from build123d import *

# Parameters (mm, degrees)
BOSS_EXTRUDE1_DEPTH = 6


with BuildPart() as part:
    # Sketch1 → Boss-Extrude1 (new body)
    with BuildSketch(Plane.XY):
        Polygon((20, -35), (20, 35), (10, 45), (10, 51), (-10, 51), (-10, 45), (-20, 35), (-20, -35), (-10, -45), (-10, -51), (10, -51), (10, -45), align=None)
        Polygon((5.757359313, 40.757359313), (15.757359313, 30.757359313), (15.757359313, -30.757359313), (5.757359313, -40.757359313), (-5.757359313, -40.757359313), (-15.757359313, -30.757359313), (-15.757359313, 30.757359313), (-5.757359313, 40.757359313), align=None, mode=Mode.SUBTRACT)
    extrude(amount=BOSS_EXTRUDE1_DEPTH)


solid = part.part
Check sheet for the modelled part. Datum: model origin and axes. Units: mm. A direction names the side the tool comes from. Give positions to 0.01 mm unless a question says otherwise; leave off trailing zeros. Write each loop counter-clockwise with the first axis right and the second up, starting at its lowest first coordinate (ties: lowest second). Pieces come first, ordered by that corner, then holes. Notation, with made-up numbers: (34, -36.75) -> (40, -36.75) arc R6 ccw to (40, -26.75) -> close; hole circle Ø6 at (70.25, 84.25). An arc over 180 degrees is marked (long way). Use one line per item in the form item = value. Start each with the question number.
1. Access from +Z, -Z, +X, -X, +Y, -Y to the whole of each face (thin tool, end or side, straight path). Record for faces 4 (the flat face through (-10, 48, 3)), 5 (the flat face through (10, 48, 3)), 6 (the flat face through (0, -51, 3)), 7 (the flat face through (-20, 0, 3)), 8 (the flat face through (-10.687, -35.827, 2.958)).
2. Section check C-C (y = 15). Record the cut outline in (x, z).
3. Section check A-A (z = 1.75). Record the cut outline in (x, y), and give its area (3 significant figures).
4. Mould release check, pull along Y, two halves, no side actions. Record for faces 1 (the flat face through (10, -48, 3)), 2 (the flat face through (-15, -40, 3)), 3 (the flat face through (15.757, 0, 3)): pulls with the +Y half, pulls with the -Y half, needs draft (parallel to the pull), parting line crosses it, or undercut.
5. Go/stop test with flat-tipped pins: P1, Ø12, axis at x = 8.5, y = -4.5, coming from the +Z side; P2, Ø1.8, axis at y = -47, z = 4.5, coming from the -X side. Record where each tip stops, or that it passes through.
6. Section check B-B (x = 3.5). Record the cut outline in (y, z), and give its area (3 significant figures).
7. Thickness scan on line 1 along Y through (x, z) = (0, 2.15); line 2 along X through (y, z) = (-14.5, 2.25); line 3 along Y through (x, z) = (-8, 5.5). Record the ranges inside material, lowest first. Write a range as from..to.
Conclusion:
q1.face_4 = +Z, -Z, -X, +Y
q1.face_5 = +Z, -Z, +X, +Y
q1.face_6 = +Z, -Z, +X, -X, -Y
q1.face_7 = +Z, -Z, -X, +Y, -Y
q1.face_8 = +Z, -Z
q2.outline = (-20, 0) -> (-15.76, 0) -> (-15.76, 6) -> (-20, 6) -> close; (15.76, 0) -> (20, 0) -> (20, 6) -> (15.76, 6) -> close
q3.outline = (-20, -35) -> (-10, -45) -> (-10, -51) -> (10, -51) -> (10, -45) -> (20, -35) -> (20, 35) -> (10, 45) -> (10, 51) -> (-10, 51) -> (-10, 45) -> (-20, 35) -> close; hole (-15.76, -30.76) -> (-5.76, -40.76) -> (5.76, -40.76) -> (15.76, -30.76) -> (15.76, 30.76) -> (5.76, 40.76) -> (-5.76, 40.76) -> (-15.76, 30.76) -> close
q3.area = 1,270 mm²
q4.face_1 = needs draft
q4.face_2 = pulls with the -Y half
q4.face_3 = undercut
q5.P1 = through
q5.P2 = -10
q6.outline = (-51, 0) -> (-40.76, 0) -> (-40.76, 6) -> (-51, 6) -> close; (40.76, 0) -> (51, 0) -> (51, 6) -> (40.76, 6) -> close
q6.area = 123 mm²
q7.line_1 = -51..-40.76, 40.76..51
q7.line_2 = -20..-15.76, 15.76..20
q7.line_3 = -51..-38.51, 38.51..51
